Model file for the job. Use its own axes, mm. A direction names the side the tool comes from. Give positions to 0.01 mm unless a question says otherwise; leave off trailing zeros. Write each loop counter-clockwise with the first axis right and the second up, starting at its lowest first coordinate (ties: lowest second). Pieces come first, ordered by that corner, then holes. Notation, with made-up numbers: M 23.5,37 L 29.5,37 A29 ccw 29.5,57 Z; hole C 51,32 d2. An arc over 180 degrees is marked long. Answer as a JSON object with one key per item and string values. Group by question number.
```python
from build123d import *

# Parameters (mm, degrees)
F0_R     = 35.56
F1_DEPTH = 185.777068
F2_T     = -2.54
F3_R     = 26.32941
F4_DEPTH = 101.879455


with BuildPart() as f1:
    # F0 (on Front) → F1 (new body)
    with BuildSketch(Plane.XZ):
        Circle(F0_R)
    extrude(amount=F1_DEPTH)

    # F2
    f2_openings = [f1.faces().sort_by_distance(p)[0] for p in [
        (0, -185.777068, 0),
    ]]
    offset(amount=F2_T, openings=f2_openings)

    # F3 (on Top) → F4 (cut)
    with BuildSketch(Plane.XY):
        with Locations((0, -62.634744)):
            Circle(F3_R)
    extrude(amount=-F4_DEPTH, mode=Mode.SUBTRACT)


solid = f1.part
```
Q1. Drop flat-ended pins along their axis: P1, Ø4, axis at y = -119, z = -2.5, coming from the -X side; P2, Ø3, axis at x = 2, y = -75, coming from the +Z side; P3, Ø6, axis at y = -36.5, z = -10.5, coming from the -X side. Give the stop position or say it passes through.
Q2. Slice it at B-B, the plane z = 0. Write the cut outline in (x, y), then the cut area to 3 significant figures.
Q3. Slice it at C-C, the plane z = -28.5. Write the cut outline in (x, y).
Q4. 3-axis set-ups, long thin cutter, end or side, ignore diameter. For faces 1 (the cylindrical face through (-19.92, -45.42, -27.71)), 2 (the flat face through (0, -2.54, 0)), 3 (the flat face through (24, -185.777, -24)): which of +Z, -Z, +X, -X, +Y, -Y reach the whole face in a straight line?
Q5. Two-plate mould, pull along Z, no slides. Class faces 4 (the flat face through (0, 0, 0)), 5 (the cylindrical face through (-4.3, -92.88, 32.74)), 6 (the cylindrical face through (-4.629, -91.588, 35.257)): +Z half, -Z half, draft (parallel to the pull), parting line (faces both ways), or undercut.
Q6. Slice it at A-A, the plane x = 0. Write the cut outline in (y, z), then the cut area to 3 significant figures.
Q7. Slice it at D-D, the plane y = -146. Write the cut outline in (x, z).
Q8. Wall check: L1, parallel to Z at x = 0, y = -145.5; L2, parallel to Y at x = 10, z = 0. Give the ranges that are in metal, low to high.
Solved:
{
 "1": {"P1": "stops at x = -35.56", "P2": "stops at z = 35.56", "P3": "stops at x = -34.76"},
 "2": {"outline": "M -35.56,-185.78 L -33.02,-185.78 L -33.02,-2.54 L 33.02,-2.54 L 33.02,-185.78 L 35.56,-185.78 L 35.56,0 L -35.56,0 Z", "area": "1,110 mm²"},
 "3": {"outline": "M -21.27,-185.78 L -16.68,-185.78 L -16.68,-83.01 A26.33 cw -21.27,-78.16 Z; M -21.27,-47.11 A26.33 cw -16.68,-42.26 L -16.68,-2.54 L 16.68,-2.54 L 16.68,-42.26 A26.33 cw 21.27,-47.11 L 21.27,0 L -21.27,0 Z; M 16.68,-185.78 L 21.27,-185.78 L 21.27,-78.16 A26.33 cw 16.68,-83.01 Z"},
 "4": {"face 1": "-Z", "face 2": "-Y", "face 3": "+Z, -Z, +X, -X, -Y"},
 "5": {"face 4": "draft", "face 5": "undercut", "face 6": "parting line"},
 "6": {"outline": "M -185.78,-35.56 L -88.96,-35.56 L -88.96,-33.02 L -185.78,-33.02 Z; M -185.78,33.02 L -2.54,33.02 L -2.54,-33.02 L -36.31,-33.02 L -36.31,-35.56 L 0,-35.56 L 0,35.56 L -185.78,35.56 Z", "area": "978 mm²"},
 "7": {"outline": "C 0,0 d71.12; hole C 0,0 d66.04"},
 "8": {"L1": "z = -35.56 to -33.02, 33.02 to 35.56", "L2": "y = -2.54 to 0"}
}
